Read the model definition and answer for the solid it produces. Units are mm, in the model's axes. A direction names the side the tool comes from. Give positions to 0.01 mm unless a question says otherwise; leave off trailing zeros. Write each loop counter-clockwise with the first axis right and the second up, starting at its lowest first coordinate (ties: lowest second). Pieces come first, ordered by that corner, then holes. Notation, with made-up numbers: (-9.75, 36) - (6.25, 36) arc R22 cw to (6.25, 72) - close; hole circle Ø6 at (17.25, 71). An arc over 180 degrees is marked (long way). Use CSV: the item, a comma, the result in double quotes. Start each with the question number.
Autodesk Fusion 360 part; units mm, degrees
sketch "Sketch1" plane through (0, 0, 0) normal (0, 0, 1) x (1, 0, 0)
  circle A0 centre (0, 0) radius 65
  circle A1 centre (0, 0) radius 61.375 construction
  circle A2 centre (0, 61.375) radius 1.5
  circle A3 centre (0, 0) radius 42.5
  dimension "d1" = 130
  dimension "d2" = 122.75
  dimension "d3" = 3
  dimension "LargeBearingDia" = 85
extrude "Extrude1" add sketch "Sketch1" along normal blind 10 contours A0 | A2
extrude "Extrude2" cut sketch "Sketch1" along normal blind 7 contours A2
pattern_circular "C-Pattern1" count 6 over 360 about axis through (0, 0, 1.75) along (0, 0, 1) of "Extrude2"
sketch "Sketch2" plane through (0, 0, 10) normal (0, 0, 1) x (-1, 0, 0)
  circle A0 centre (0, 0) radius 42.5
  circle A1 centre (0, 0) radius 65
  circle A2 centre (0, 0) radius 52.5 construction
  circle A3 centre (0, -52.5) radius 7.05
  circle A4 centre (28.3836, -44.1658) radius 7.05
  circle A5 centre (47.7557, -21.8093) radius 7.05
  circle A6 centre (51.9656, 7.4715) radius 7.05
  circle A7 centre (39.6769, 34.3802) radius 7.05
  circle A8 centre (14.791, 50.3734) radius 7.05
  circle A9 centre (-14.791, 50.3734) radius 7.05
  circle A10 centre (-39.6769, 34.3802) radius 7.05
  circle A11 centre (-51.9656, 7.4715) radius 7.05
  circle A12 centre (-47.7557, -21.8093) radius 7.05
  circle A13 centre (-28.3836, -44.1658) radius 7.05
  circle A14 centre (0, 0) radius 56.5
  dimension "d11" = 105
  dimension "d12" = 14.1
  dimension "d14" = 360
  dimension "d15" = 113
extrude "Extrude3" add sketch "Sketch2" along normal blind 17.5 contours A1
extrude "Extrude4" add 1 faces at (57.7924, -22.5756, 27.5) along direction (0, 0, 1) blind 1.75
sketch "Sketch3" plane through (0, 0, 29.25) normal (0, 0, 1) x (-1, 0, 0)
  arc A0 (53.6005, -17.8672) -> (56.4631, 2.0424) centre (0, 0) ccw
  arc A1 (48.604, -28.8081) -> (53.6005, -17.8672) centre (47.7557, -21.8093) ccw
  arc A2 (35.4319, -44.0094) -> (48.604, -28.8081) centre (0, 0) ccw
  arc A3 (25.3134, -50.5122) -> (35.4319, -44.0094) centre (28.3836, -44.1658) ccw
  arc A4 (6.0139, -56.179) -> (25.3134, -50.5122) centre (0, 0) ccw
  arc A5 (-6.0139, -56.179) -> (6.0139, -56.179) centre (0, -52.5) ccw
  arc A6 (-25.3134, -50.5122) -> (-6.0139, -56.179) centre (0, 0) ccw
  arc A7 (-35.4319, -44.0094) -> (-25.3134, -50.5122) centre (-28.3836, -44.1658) ccw
  arc A8 (-48.604, -28.8081) -> (-35.4319, -44.0094) centre (0, 0) ccw
  arc A9 (-53.6005, -17.8672) -> (-48.604, -28.8081) centre (-47.7557, -21.8093) ccw
  arc A10 (-56.4631, 2.0424) -> (-53.6005, -17.8672) centre (0, 0) ccw
  arc A11 (-54.7513, 13.9478) -> (-56.4631, 2.0424) centre (-51.9656, 7.4715) ccw
  arc A12 (-46.3956, 32.2444) -> (-54.7513, 13.9478) centre (0, 0) ccw
  arc A13 (-38.519, 41.3345) -> (-46.3956, 32.2444) centre (-39.6769, 34.3802) ccw
  arc A14 (-21.5978, 52.2091) -> (-38.519, 41.3345) centre (0, 0) ccw
  arc A15 (-10.0571, 55.5977) -> (-21.5978, 52.2091) centre (-14.791, 50.3734) ccw
  arc A16 (10.0571, 55.5977) -> (-10.0571, 55.5977) centre (0, 0) ccw
  arc A17 (21.5978, 52.2091) -> (10.0571, 55.5977) centre (14.791, 50.3734) ccw
  arc A18 (38.519, 41.3345) -> (21.5978, 52.2091) centre (0, 0) ccw
  arc A19 (46.3956, 32.2444) -> (38.519, 41.3345) centre (39.6769, 34.3802) ccw
  arc A20 (54.7513, 13.9478) -> (46.3956, 32.2444) centre (0, 0) ccw
  arc A21 (56.4631, 2.0424) -> (54.7513, 13.9478) centre (51.9656, 7.4715) ccw
  circle A22 centre (0, 0) radius 65
  circle A23 centre (0, 0) radius 61.0224 construction
  circle A24 centre (0, -61.0224) radius 1.5
  circle A25 centre (52.847, -30.5112) radius 1.5
  circle A26 centre (52.847, 30.5112) radius 1.5
  circle A27 centre (0, 61.0224) radius 1.5
  circle A28 centre (-52.847, 30.5112) radius 1.5
  circle A29 centre (-52.847, -30.5112) radius 1.5
  dimension "d20" = 3
  dimension "d22" = 360
  dimension "d25" = 122.0449
extrude "Extrude5" cut sketch "Sketch3" against normal blind 10 contours A5 A24 | A25 | A26 | A27 | A28 | A29 picked at (-0.1447, -59.5399)
equation "d3 = ScrewDia_3mm"
equation "d20 = ScrewDia_3mm"
equation "ScrewDia_3mm = 3 mm"
(1) Which of the six approach directions +Z, -Z, +X, -X, +Y, -Y give full straight-line access (tool end or side, diameter ignored) to faces 1 (the face through (42, -14, 0)), 2 (the face through (-52.957, 32.175, 3.451)), 3 (the face through (-54.23, 31.09, 24.32))?
(2) The part is cut by section B-B on x = -32. Write down the section's boundary in (y, z).
(3) Given P1, Ø0.9, axis at x = 53.5, y = 31, coming from the -Z side; P2, Ø2, axis at x = 16, y = -39.5, coming from the +Z side; P3, Ø1.5, axis at y = -47, z = 19, coming from the +X side; P4, Ø2.5, axis at x = -52, y = -31, coming from the +Z side, each flat-ended and moving along its own axis, determine where each tip first touches the part or whether it passes through.
(4) The part is cut by section A-A on y = 40. Write down the section's boundary in (x, z), plus the area to 3 significant figures.
(5) For a pull along X with two mould halves and no side action, classify faces 4 (the face through (53, 31, 7)), 5 (the face through (53.3, -19.6, 29.25)) as pulls with the +X half, pulls with the -X half, needs draft (parallel to the pull), parting line crosses it, or undercut.
(6) The part is cut by section C-C on z = 24.25. Write down the section's boundary in (x, y), plus the area to 3 significant figures.
(7) Consider probe 1 along Y at (x, z) = (0, 3) (3 decimals); probe 2 along Y at (x, z) = (-0.5, 24.75); probe 3 along Z at (x, y) = (-51, -22.5). Determine where each line is inside the solid, lowest interval first.
Reported:
1,face 1,"-Z, +X, -X, +Y, -Y"
1,face 2,"-Z"
1,face 3,"+Z"
2,outline,"(-56.58, 0) - (-27.97, 0) - (-27.97, 10) - (-46.56, 10) - (-46.56, 29.25) - (-56.58, 29.25) - close; (27.97, 0) - (56.58, 0) - (56.58, 29.25) - (50.22, 29.25) - (50.22, 10) - (27.97, 10) - close"
3,P1,"z = 7"
3,P2,"z = 10"
3,P3,"x = 45.67"
3,P4,"z = 29.25"
4,outline,"(-51.23, 0) - (-14.36, 0) - (-14.36, 10) - (-39.9, 10) - (-39.9, 29.25) - (-51.23, 29.25) - close; (14.36, 0) - (51.23, 0) - (51.23, 29.25) - (39.9, 29.25) - (39.9, 10) - (14.36, 10) - close"
4,area,"1,170 mm²"
5,face 4,"undercut"
5,face 5,"needs draft"
6,outline,"circle Ø130 at (0, 0); hole (-56.46, -2.04) arc R7.05 ccw to (-54.75, -13.95) arc R56.5 ccw to (-46.4, -32.24) arc R7.05 ccw to (-38.52, -41.33) arc R56.5 ccw to (-21.6, -52.21) arc R7.05 ccw to (-10.06, -55.6) arc R56.5 ccw to (10.06, -55.6) arc R7.05 ccw to (21.6, -52.21) arc R56.5 ccw to (38.52, -41.33) arc R7.05 ccw to (46.4, -32.24) arc R56.5 ccw to (54.75, -13.95) arc R7.05 ccw to (56.46, -2.04) arc R56.5 ccw to (53.6, 17.87) arc R7.05 ccw to (48.6, 28.81) arc R56.5 ccw to (35.43, 44.01) arc R7.05 ccw to (25.31, 50.51) arc R56.5 ccw to (6.01, 56.18) arc R7.05 ccw to (-6.01, 56.18) arc R56.5 ccw to (-25.31, 50.51) arc R7.05 ccw to (-35.43, 44.01) arc R56.5 ccw to (-48.6, 28.81) arc R7.05 ccw to (-53.6, 17.87) arc R56.5 ccw to start; hole circle Ø3 at (-52.85, -30.51); hole circle Ø3 at (-52.85, 30.51); hole circle Ø3 at (0, -61.02); hole circle Ø3 at (52.85, -30.51); hole circle Ø3 at (52.85, 30.51)"
6,area,"2,920 mm²"
7,probe 1,"-65 to -62.875, -59.875 to -42.5, 42.5 to 59.875, 62.875 to 65"
7,probe 2,"-65 to -62.44, -59.61 to -56.5, 59.53 to 65"
7,probe 3,"0 to 10"
